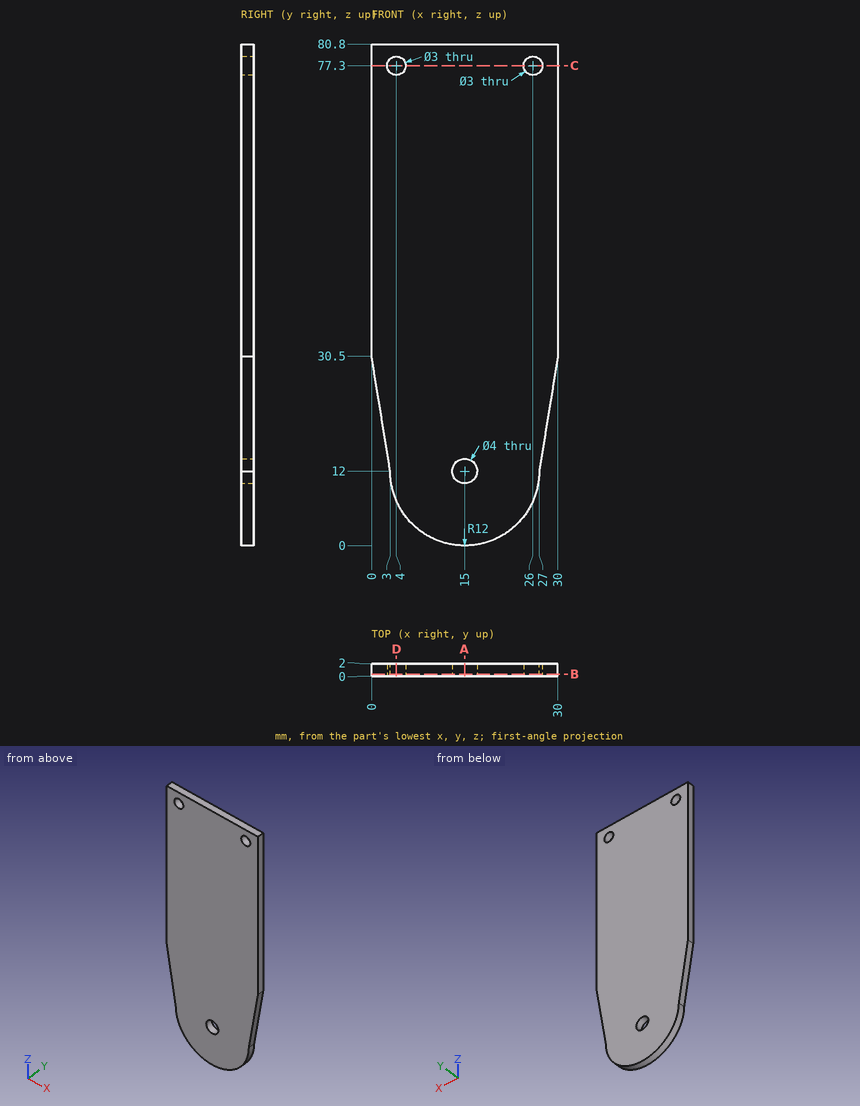
The drawing under review shows one solid part. Ordinate dimensions are in mm from its lowest x, y, z. Round coordinates to 2 decimals unless told otherwise and drop trailing zeros. Write each loop counter-clockwise with the first axis right and the second up, starting at its lowest first coordinate (ties: lowest second). Pieces come first, ordered by that corner, then holes. Notation, with made-up numbers: (88.25, -30) -> (147.25, -30) arc R27 cw to (147.25, -8) -> close; hole circle Ø3 at (-9.75, 13.5). An arc over 180 degrees is marked (long way). One line per question, with ' | ' between items.
(1) Take a section at C-C, the plane z = 77.3. State the section outline as (x, y) points, and give its area (3 significant figures).
Result sheet:
outline: (0, 0) -> (2.5, 0) -> (2.5, 2) -> (0, 2) -> close; (5.5, 0) -> (24.5, 0) -> (24.5, 2) -> (5.5, 2) -> close; (27.5, 0) -> (30, 0) -> (30, 2) -> (27.5, 2) -> close | area: 48.0 mm2
(2) Take a section at B-B, the plane y = 0.3. State the section outline as (x, z) points, and give its area (3 significant figures).
Result sheet:
outline: (0, 30.5) -> (3, 12) arc R12 ccw to (27, 12) -> (30, 30.5) -> (30, 80.8) -> (0, 80.8) -> close; hole circle Ø3 at (4, 77.3); hole circle Ø4 at (15, 12); hole circle Ø3 at (26, 77.3) | area: 2,210 mm2
(3) Take a section at A-A, the plane x = 15. State the section outline as (y, z) points.
Result sheet:
outline: (0, 0) -> (2, 0) -> (2, 10) -> (0, 10) -> close; (0, 14) -> (2, 14) -> (2, 80.8) -> (0, 80.8) -> close
(4) Insertion check: P1, Ø5, axis at x = 4, z = 77.3, coming from the +Y side; P2, Ø2.5, axis at x = 26, z = 77.3, coming from the +Y side. Each pin has a flat end and moves straight along its axis. Give the tip position at first contact, or say it passes through.
Result sheet:
P1: y = 2 | P2: through
(5) Wall thickness on line 1 (X direction, y = 0.75, z = 77.3); line 2 (X direction, y = 1.4, z = 12); line 3 (Z direction, x = 4.5, y = 0.55): over which ranges is each line inside the solid? List them lowest first. Write a range as [from, to].
Result sheet:
line 1: [0, 2.5], [5.5, 24.5], [27.5, 30] | line 2: [3, 13], [17, 27] | line 3: [6.19, 75.89], [78.71, 80.8]
(6) Take a section at D-D, the plane x = 4. State the section outline as (y, z) points.
Result sheet:
outline: (0, 7.2) -> (2, 7.2) -> (2, 75.8) -> (0, 75.8) -> close; (0, 78.8) -> (2, 78.8) -> (2, 80.8) -> (0, 80.8) -> close
